Geometry check sheet. Reference: the model listing, model coordinates, mm. Face numbers are marked on the shaded views. Round coordinates to 2 decimals unless told otherwise and drop trailing zeros.
```python
from build123d import *

# Parameters (mm, degrees)
SKETCH1_R                    = 34.671
SKETCH1_R_2                  = 20.6375
BOSS_EXTRUDE1_DEPTH          = 12.7
SKETCH2_R                    = 22.225
CUT_EXTRUDE1_DEPTH           = 7.3914
CHAMFER1_SIZE                = 0.762
SKETCH4_R                    = 3.3655
CUT_EXTRUDE2_DEPTH           = 13.7
CHAMFER2_SIZE                = 0.381
CIRPATTERN1_COUNT            = 6
CHAMFER2_OF_CIRPATTERN1_SIZE = 0.381
CUT_EXTRUDE3_DEPTH           = 0.79375


with BuildPart() as part:
    # Sketch1 → Boss-Extrude1 (new body)
    with BuildSketch(Plane(origin=(0, 0, 0), x_dir=(1, 0, 0), z_dir=(0, 1, 0))):
        Circle(SKETCH1_R)
        Circle(SKETCH1_R_2, mode=Mode.SUBTRACT)
    extrude(amount=BOSS_EXTRUDE1_DEPTH)

    # Sketch2 → Cut-Extrude1 (cut)
    with BuildSketch(Plane(origin=(0, 12.7, 0), x_dir=(1, 0, 0), z_dir=(0, 1, 0))):
        Circle(SKETCH2_R)
    extrude(amount=-CUT_EXTRUDE1_DEPTH, mode=Mode.SUBTRACT)

    # Chamfer1
    chamfer1_edges = [part.edges().sort_by_distance(p)[0] for p in [
        (-22.225, 12.7, 0),
        (-34.671, 0, 0),
        (-34.671, 12.7, 0),
    ]]
    chamfer(chamfer1_edges, length=CHAMFER1_SIZE)

    # Sketch3 → Cut-Revolve1 (revolve, cut)
    with BuildSketch(Plane.XY):
        Polygon((-24.1554, 0), (-24.1554, 1.825244), (-20.955, 0.6604), (-20.955, 1.27), (0, 1.27), (0, 0), align=None)
    revolve(axis=Axis((0, 12.7, 0), (0, -1, 0)), mode=Mode.SUBTRACT)

    # Sketch4 → Cut-Extrude2 (cut, through all)
    with BuildSketch(Plane(origin=(0, 12.7, 0), x_dir=(1, 0, 0), z_dir=(0, 1, 0))):
        with Locations((0, 29.3624)):
            Circle(SKETCH4_R)
    cut_extrude2 = extrude(amount=-CUT_EXTRUDE2_DEPTH, mode=Mode.SUBTRACT)

    # Chamfer2
    chamfer2_edges = [part.edges().sort_by_distance(p)[0] for p in [
        (-3.3655, 0, -29.3624),
        (-3.3655, 12.7, -29.3624),
    ]]
    chamfer(chamfer2_edges, length=CHAMFER2_SIZE)

    # CirPattern1: Cut-Extrude2 ×6 about axis
    cirpattern1_axis = Axis((0, 0, 0), (0, 1, 0))
    for i in range(1, CIRPATTERN1_COUNT):
        add(cut_extrude2.rotate(cirpattern1_axis, i * 360 / CIRPATTERN1_COUNT), mode=Mode.SUBTRACT)

    # Chamfer2 of CirPattern1
    chamfer2_of_cirpattern1_edges = [part.edges().sort_by_distance(p)[0] for p in [
        (-27.111334316, 0, -11.766591504),
        (-27.111334316, 12.7, -11.766591504),
        (-23.745834316, 0, 17.595808496),
        (-23.745834316, 12.7, 17.595808496),
        (3.3655, 0, 29.3624),
        (3.3655, 12.7, 29.3624),
        (27.111334316, 0, 11.766591504),
        (27.111334316, 12.7, 11.766591504),
        (23.745834316, 0, -17.595808496),
        (23.745834316, 12.7, -17.595808496),
    ]]
    chamfer(chamfer2_of_cirpattern1_edges, length=CHAMFER2_OF_CIRPATTERN1_SIZE)

    # Sketch5 → Cut-Extrude3 (cut, symmetric)
    with BuildSketch(Plane.XY):
        Polygon((-23.765182704, 0.94596365), (-35.869388854, 1.580318214), (-35.869388854, -0.2995168), (-23.765182704, -0.2995168), align=None)
        Polygon((23.765182704, 0.94596365), (23.765182704, -0.2995168), (35.869388854, -0.2995168), (35.869388854, 1.580318214), align=None)
    extrude(amount=CUT_EXTRUDE3_DEPTH, both=True, mode=Mode.SUBTRACT)


solid = part.part
```
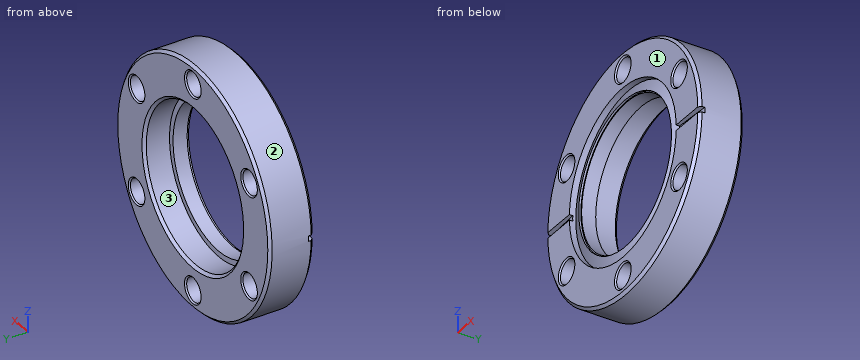
(1) Depth check by flat-ended pin: P1, Ø3, axis at y = 5, z = -7, coming from the +X side; P2, Ø22, axis at x = -8.5, z = 6.5, coming from the +Y side; P3, Ø5.5, axis at x = -25.43, z = 14.68, coming from the -Y side; P4, Ø0.5, axis at x = 32, y = 1, coming from the -Z side. Enter the tip coordinate at first touch or a pass-through.
Returned:
P1: stops at x = 34.23
P2: stops at y = 5.31
P3: passes through
P4: stops at z = -13.93
(2) Material ranges on line 1 (Z direction, x = 0, y = 7.75) (3 decimals); line 2 (Z direction, x = 25.5, y = 4); line 3 (Z direction, x = -25, y = 11.5), recorded low to high.
Returned:
line 1: z = -34.671 to -32.728, -25.997 to -22.225, 22.225 to 25.997, 32.728 to 34.671
line 2: z = -23.49 to -18.05, -11.32 to 11.32, 18.05 to 23.49
line 3: z = -24.02 to -18.02, -11.34 to 11.34, 18.02 to 24.02
(3) Draft check along X on the marked faces 1, 2 and 3. Enter one of: released by +X, released by -X, zero draft, split by the parting line, or undercut.
Returned:
face 1: zero draft
face 2: split by the parting line
face 3: undercut
(4) Sectioned sample at B-B, the plane x = 0. Give the number of separate pieces and of enclosed holes in the cut face, and give its area (3 significant figures).
Returned:
separate pieces: 4
enclosed holes: 0
area: 151 mm2
